from build123d import *

# Parameters (mm, degrees)
SKETCH_1_R          = 5.25
SKETCH_1_R_2        = 2.25
EXTRUDE_1_DEPTH     = 22.2
SKETCH_2_W          = 16
SKETCH_2_H          = 9
EXTRUDE_2_DEPTH     = 22.2
SKETCH_3_W          = 12
SKETCH_3_H          = 5.4
CUT_EXTRUDE_1_DEPTH = 30.370946529
SKETCH_4_R          = 1.65
CUT_EXTRUDE_2_DEPTH = 22


with BuildPart() as part:
    # 草图1 → 凸台-拉伸1 (new body)
    with BuildSketch(Plane(origin=(0, 0, 0), x_dir=(1, 0, 0), z_dir=(0, 1, 0))):
        with Locations(Location((0, 0, 0), (0, 0, 270))):
            Circle(SKETCH_1_R)
        with Locations(Location((0, 0, 0), (0, 0, 270))):
            Circle(SKETCH_1_R_2, mode=Mode.SUBTRACT)
    extrude(amount=EXTRUDE_1_DEPTH)

    # 草图2 → 凸台-拉伸2 (add)
    with BuildSketch(Plane(origin=(0, 22.2, 0), x_dir=(1, 0, 0), z_dir=(0, 1, 0))):
        with Locations((10.5, 0)):
            Rectangle(SKETCH_2_W, SKETCH_2_H)
    extrude(amount=-EXTRUDE_2_DEPTH)

    # 草图3 → 切除-拉伸1 (cut, through all)
    with BuildSketch(Plane(origin=(0, 22.2, 0), x_dir=(1, 0, 0), z_dir=(0, 1, 0))):
        with Locations((12.5, 0)):
            Rectangle(SKETCH_3_W, SKETCH_3_H)
    extrude(amount=-CUT_EXTRUDE_1_DEPTH, mode=Mode.SUBTRACT)

    # 草图4 → 切除-拉伸2 (cut)
    with BuildSketch(Plane.XY.offset(4.5)):
        with Locations(Location((12.5, 15.1, 0), (0, 0, 180))):
            Circle(SKETCH_4_R)
        with Locations(Location((12.5, 7.1, 0), (0, 0, 180))):
            Circle(SKETCH_4_R)
    extrude(amount=-CUT_EXTRUDE_2_DEPTH, mode=Mode.SUBTRACT)


solid = part.part
The listing builds one solid part. Answer for the finished solid, in the listing's coordinates (mm). A direction names the side the tool comes from. Give positions to 0.01 mm unless a question says otherwise; leave off trailing zeros. Write each loop counter-clockwise with the first axis right and the second up, starting at its lowest first coordinate (ties: lowest second). Pieces come first, ordered by that corner, then holes.
Item 1: Section D-D, the plane x = 9.5 is taken. Write down the section's boundary in (y, z), plus the area to 3 significant figures.
Item 2: Section C-C, the plane z = -0.75 is taken. Write down the section's boundary in (x, y).
Item 3: Section B-B, the plane x = 12.5 is taken. Write down the section's boundary in (y, z).
Item 4: Determine the mould class of faces 5 (the cylindrical face through (0.676, 10.945, 2.146)), 6 (the flat face through (4, 22.2, 0)), 7 (the cylindrical face through (10.976, 7.732, -3.587)) for opening direction Y: released by +Y, released by -Y, zero draft, split by the parting line, or undercut.
Item 5: Flat-ended cylindrical pins translate along their axes: P1, Ø6, axis at x = 14.5, z = -1.5, coming from the -Y side; P2, Ø9.5, axis at x = 15.5, y = 6, coming from the +Z side; P3, Ø1, axis at y = 6.5, z = 0, coming from the +X side; P4, Ø3, axis at x = 9, y = 8, coming from the -Z side. Find the tip coordinate at first contact, or state that the pin passes through.
Item 6: Find the intervals of material crossed by line 1 along Y through (x, z) = (12.5, 3.9); line 2 along Z through (x, y) = (13.25, 17.75); line 3 along Y through (x, z) = (13.25, -3), in increasing order.
Item 7: Which of the six approach directions +Z, -Z, +X, -X, +Y, -Y give full straight-line access (tool end or side, diameter ignored) to faces 1 (the flat face through (10, 11, 4.5)), 2 (the flat face through (10, 11, -4.5)), 3 (the flat face through (12, 11, -2.7)), 4 (the cylindrical face through (10.976, 15.732, 3.613))?
Item 8: Section A-A, the plane y = 15.1 is taken. Write down the section's boundary in (x, z).
Completed:
1. outline: (0, -4.5) - (22.2, -4.5) - (22.2, -2.7) - (0, -2.7) - close; (0, 2.7) - (22.2, 2.7) - (22.2, 4.5) - (0, 4.5) - close
1. area: 79.9 mm2
2. outline: (-5.2, 0) - (-2.12, 0) - (-2.12, 22.2) - (-5.2, 22.2) - close; (2.12, 0) - (6.5, 0) - (6.5, 22.2) - (2.12, 22.2) - close
3. outline: (0, -4.5) - (5.45, -4.5) - (5.45, -2.7) - (0, -2.7) - close; (0, 2.7) - (5.45, 2.7) - (5.45, 4.5) - (0, 4.5) - close; (8.75, -4.5) - (13.45, -4.5) - (13.45, -2.7) - (8.75, -2.7) - close; (8.75, 2.7) - (13.45, 2.7) - (13.45, 4.5) - (8.75, 4.5) - close; (16.75, -4.5) - (22.2, -4.5) - (22.2, -2.7) - (16.75, -2.7) - close; (16.75, 2.7) - (22.2, 2.7) - (22.2, 4.5) - (16.75, 4.5) - close
4. face 5: zero draft
4. face 6: released by +Y
4. face 7: undercut
5. P1: stops at y = 0
5. P2: stops at z = 4.5
5. P3: stops at x = 6.5
5. P4: stops at z = -4.5
6. line 1: y = 0 to 5.45, 8.75 to 13.45, 16.75 to 22.2
6. line 2: z = -4.5 to -2.7, 2.7 to 4.5
6. line 3: y = 0 to 5.63, 8.57 to 13.63, 16.57 to 22.2
7. face 1: +Z, +X, +Y, -Y
7. face 2: -Z, +X, +Y, -Y
7. face 3: +X, +Y, -Y
7. face 4: +Z, -Z
8. outline: (2.7, -4.5) - (10.85, -4.5) - (10.85, -2.7) - (6.5, -2.7) - (6.5, 2.7) - (10.85, 2.7) - (10.85, 4.5) - (2.7, 4.5) arc R5.25 ccw (long way) to start; (14.15, -4.5) - (18.5, -4.5) - (18.5, -2.7) - (14.15, -2.7) - close; (14.15, 2.7) - (18.5, 2.7) - (18.5, 4.5) - (14.15, 4.5) - close; hole circle Ø4.5 at (0, 0)
